Input: dimensioned drawing with shaded views. Units: mm. Origin: part minimum x, y, z. Coordinates: 2 decimals unless noted, no trailing zeros. Loops run counter-clockwise (first coordinate to the right, second up) from the corner with the lowest first, then second, coordinate; pieces in that order, holes last.
(1) Section B-B, the plane y = 0.5. Give the number of separate pieces and of enclosed holes in the cut face, then the cut area to 3 significant figures.
(2) Section A-A, the plane z = 6.35. Return loops of the section in (x, y), then the cut area to 3 significant figures.
(3) Section C-C, the plane z = 2.5. Return loops of the section in (x, y).
(4) Line query: L1, parallel to X at y = 2.75, z = 6.35; L2, parallel to X at y = 0.7, z = 3. Output: solid intervals per line, ascending.
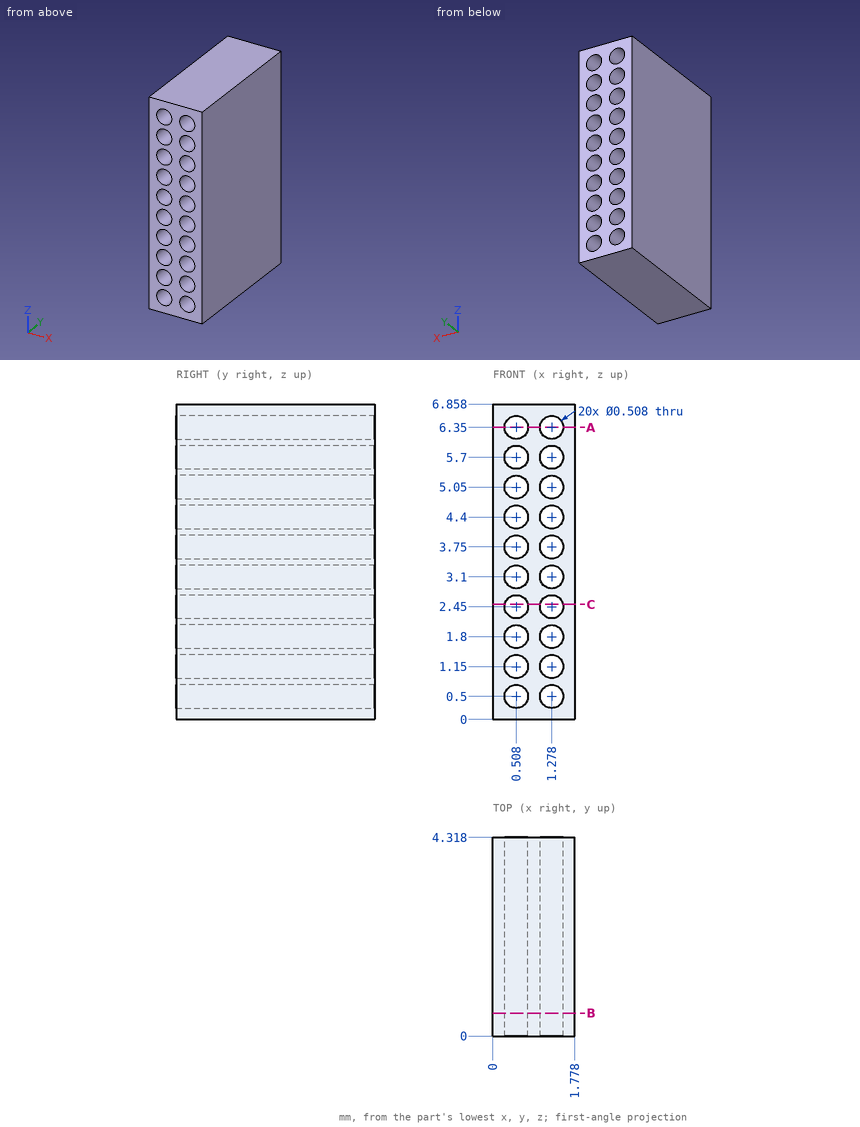
Report:
1. separate pieces: 1
1. enclosed holes: 20
1. area: 8.14 mm2
2. outline: (0, 0) - (0.25, 0) - (0.25, 4.32) - (0, 4.32) - close; (0.76, 0) - (1.02, 0) - (1.02, 4.32) - (0.76, 4.32) - close; (1.53, 0) - (1.78, 0) - (1.78, 4.32) - (1.53, 4.32) - close
2. area: 3.29 mm2
3. outline: (0, 0) - (0.26, 0) - (0.26, 4.32) - (0, 4.32) - close; (0.76, 0) - (1.03, 0) - (1.03, 4.32) - (0.76, 4.32) - close; (1.53, 0) - (1.78, 0) - (1.78, 4.32) - (1.53, 4.32) - close
4. L1: x = 0 to 0.25, 0.76 to 1.02, 1.53 to 1.78
4. L2: x = 0 to 0.27, 0.74 to 1.04, 1.51 to 1.78
